from build123d import *

# Parameters (mm, degrees)
F0_W        = 83.7067794055
F0_H        = 45.5432236195
F1_DEPTH    = 61.976
F2_T1_DEPTH = 336.3431931548
F3_T        = -12.7


# Not quite as in the source:
# - a fillet or chamfer that OpenCascade refuses, or shapes differently, is made with other operations: its cross-section is extruded or revolved along the edge and cut away or added


with BuildPart() as f1:
    # F0 (on Top) → F1 (new body)
    with BuildSketch(Plane.XY):
        with Locations((11.8514457718, -7.8249704093)):
            Rectangle(F0_W, F0_H)
    extrude(amount=F1_DEPTH)

    # F2: fillet of radius 50.8 on 1 edges, made by hand

    # F2_s2 → F2_t1 (cut)
    with BuildSketch(Plane.YZ.offset(-156.3201508057)):
        with BuildLine():
            ThreePointArc((-30.596582219, 11.4487172501), (-17.5304147843, 45.4604487546), (14.9466414005, 61.976))
            Line((14.9466414005, 61.976), (-30.596582219, 61.976))
            Line((-30.596582219, 61.976), (-30.596582219, 11.4487172501))
        make_face()
    extrude(amount=F2_T1_DEPTH, mode=Mode.SUBTRACT)

    # F3
    f3_openings = [f1.faces().sort_by_distance(p)[0] for p in [
        (11.851446, 14.946641, 30.988),
        (11.851446, -7.82497, 0),
    ]]
    offset(amount=F3_T, openings=f3_openings)

    # F4: F1 across face


with BuildPart() as f1_1:
    add(f1.part)
    add(f1.part.mirror(Plane(origin=(11.8514457718, 14.9466414005, 38.893861799), x_dir=(-1, 0, 0), z_dir=(0, 1, 0))))


solid = f1_1.part
Model file for the job. Use its own axes, mm. A direction names the side the tool comes from. Give positions to 0.01 mm unless a question says otherwise; leave off trailing zeros. Write each loop counter-clockwise with the first axis right and the second up, starting at its lowest first coordinate (ties: lowest second). Pieces come first, ordered by that corner, then holes. Notation, with made-up numbers: M 81,50 L 135,50 A21 ccw 135,69 Z; hole C -28,62 d11. An arc over 180 degrees is marked long. One line per item, written item: value. Start each with the question number.
Q1. Probe probe 1 along Y at (x, z) = (-11, 5.5); probe 2 along X at (y, z) = (19, 41); probe 3 along Y at (x, z) = (17.5, 14.5). List the from-to ranges inside material, lowest first. Write a range as [from, to].
Q2. Saw through at A-A, the plane z = 9. Write the cut outline in (x, y), plus the area to 3 significant figures.
Q3. Saw through at D-D, the plane z = 24.5. Write the cut outline in (x, y), plus the area to 3 significant figures.
Q4. 3-axis set-ups, long thin cutter, end or side, ignore diameter. For faces 1 (the flat face through (11, 47.79, 6)), 2 (the flat face through (11, 60.49, 6)): which of +Z, -Z, +X, -X, +Y, -Y reach the whole face in a straight line?
Q5. Drop flat-ended pins along their axis: pin 1 Ø8 at (x, y) = (-5, -8.5) entering from -Z; pin 2 Ø3 at (x, z) = (36, 31.5) entering from -Y; pin 3 Ø1.5 at (x, z) = (22, 19) entering from +Y. Give the stop position or say it passes through.
Q6. Saw through at C-C, the plane y = -16. Write the cut outline in (x, z).
Q7. Saw through at B-B, the plane x = 15.5. Write the cut outline in (y, z), plus the area to 3 significant figures.
Q8. Two-plate mould, pull along X, no slides. Class faces 3 (the flat face through (41.005, 15, 19)), 4 (the flat face through (53.705, 16, 24)), 5 (the cylindrical face through (11.27, 47.77, 45.07)): +X half, -X half, draft (parallel to the pull), parting line (faces both ways), or undercut.
Output values:
1. probe 1: y = [-30.6, -17.9], [47.79, 60.49]
1. probe 2: x = [-30, -17.3], [41, 53.7]
1. probe 3: y = [-30.5, -17.77], [47.67, 60.4]
2. outline: M -30,-30.6 L 53.7,-30.6 L 53.7,60.49 L -30,60.49 Z; hole M -17.3,-17.9 L 41,-17.9 L 41,47.79 L -17.3,47.79 Z
2. area: 3,790 mm²
3. outline: M -30,-28.89 L 53.7,-28.89 L 53.7,58.78 L -30,58.78 Z; hole M -17.3,-15.59 L 41,-15.59 L 41,45.48 L -17.3,45.48 Z
3. area: 3,780 mm²
4. face 1: -Z
4. face 2: +Z, -Z, +X, -X, +Y
5. pin 1: stops at z = 31
5. pin 2: stops at y = -27.09
5. pin 3: stops at y = 60.03
6. outline: M -30,0 L -17.3,0 L -17.3,23.32 L 41,23.32 L 41,0 L 53.7,0 L 53.7,47.09 L -30,47.09 Z
7. outline: M -30.6,0 L -17.9,0 L -17.9,11.45 A38.1 cw 14.95,49.18 A38.1 cw 47.79,11.45 L 47.79,0 L 60.49,0 L 60.49,11.45 A50.8 ccw 14.95,61.98 A50.8 ccw -30.6,11.45 Z
7. area: 1,930 mm²
8. face 3: undercut
8. face 4: +X half
8. face 5: draft
